Part print with two shaded views. Sizes in mm from the minimum x, y, z corner. Round coordinates to 2 decimals unless told otherwise and drop trailing zeros. Write each loop counter-clockwise with the first axis right and the second up, starting at its lowest first coordinate (ties: lowest second). Pieces come first, ordered by that corner, then holes. Notation, with made-up numbers: (35, -5) -> (88, -5) arc R29 cw to (88, 17) -> close; hole circle Ø10 at (45, 31). An arc over 180 degrees is marked (long way). Answer in a Markdown table with one row per item. Add a question column.
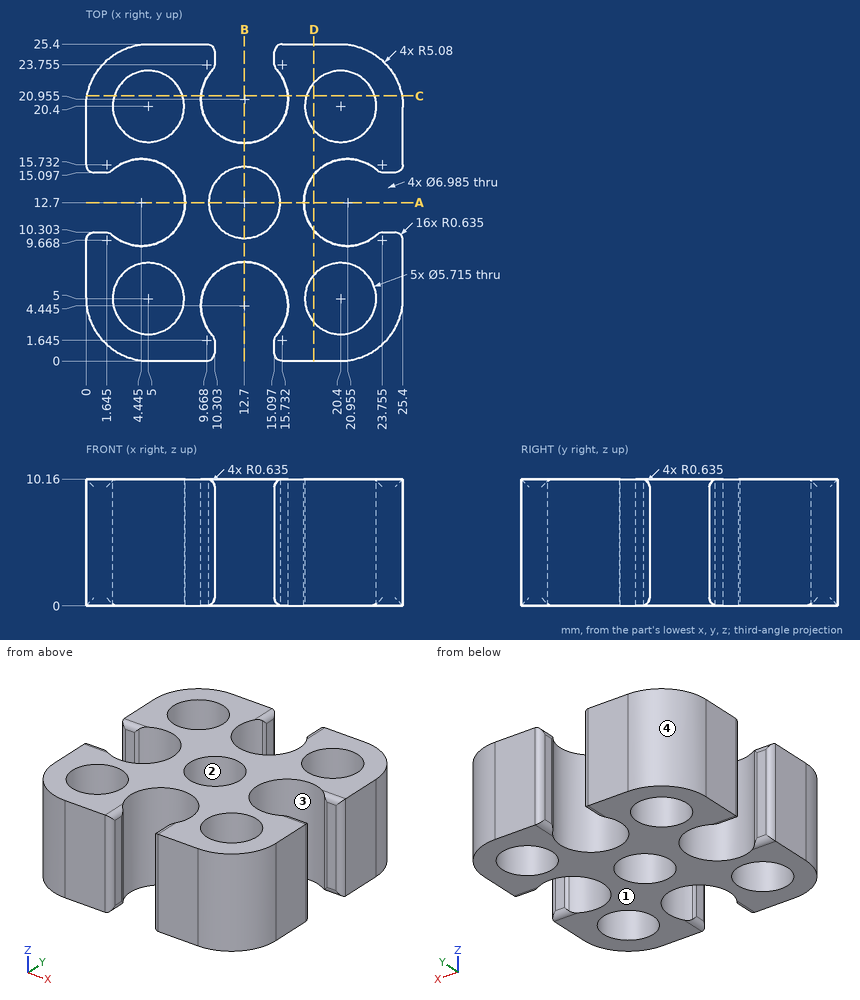
Item 1: Saw through at A-A on y = 12.7. Give the cut face in (x, z).
Item 2: Pin check, flat tips, straight feed: pin 1 (1.1 mm diameter, centred on y = 24.5, z = 6.5, fed in from +X) (1 decimal); pin 2 (11 mm diameter, centred on x = 12.7, y = 20.955, fed in from +Z); pin 3 (0.5 mm diameter, centred on y = 24, z = 5.5, fed in from -X); pin 4 (0.5 mm diameter, centred on x = 1, z = 7, fed in from +Y). Stop position of each tip, or through.
Item 3: Saw through at C-C on y = 21.25. Give the cut face in (x, z) (1 decimal).
Item 4: Saw through at D-D on x = 18.25. Give the cut face in (y, z).
Item 5: Drill centre lines: probe 1 along X at (y, z) = (3.75, 3.25); probe 2 along X at (y, z) = (21.25, 3.75) (1 decimal). Where is each one in solid material? Low to high.
Item 6: Two-plate mould, pull along X, no slides. Class the marked faces 1, 2, 3 and 4: +X half, -X half, draft (parallel to the pull), parting line (faces both ways), or undercut.
Recorded:
| question | item | result |
|---|---|---|
| 1 | outline | (7.94, 0) -> (9.84, 0) -> (9.84, 10.16) -> (7.94, 10.16) -> close; (15.56, 0) -> (17.46, 0) -> (17.46, 10.16) -> (15.56, 10.16) -> close |
| 2 | pin 1 | x = 23.9 |
| 2 | pin 2 | z = 10.16 |
| 2 | pin 3 | x = 1.33 |
| 2 | pin 4 | y = 23.66 |
| 3 | outline | (0.1, 0) -> (2.3, 0) -> (2.3, 10.2) -> (0.1, 10.2) -> close; (7.7, 0) -> (9.2, 0) -> (9.2, 10.2) -> (7.7, 10.2) -> close; (16.2, 0) -> (17.7, 0) -> (17.7, 10.2) -> (16.2, 10.2) -> close; (23.1, 0) -> (25.3, 0) -> (25.3, 10.2) -> (23.1, 10.2) -> close |
| 4 | outline | (0, 0) -> (3.12, 0) -> (3.12, 10.16) -> (0, 10.16) -> close; (6.88, 0) -> (10.49, 0) -> (10.49, 10.16) -> (6.88, 10.16) -> close; (14.91, 0) -> (18.52, 0) -> (18.52, 10.16) -> (14.91, 10.16) -> close; (22.28, 0) -> (25.4, 0) -> (25.4, 10.16) -> (22.28, 10.16) -> close |
| 5 | probe 1 | 0.18 to 2.43, 7.57 to 9.28, 16.12 to 17.83, 22.97 to 25.22 |
| 5 | probe 2 | 0.1 to 2.3, 7.7 to 9.2, 16.2 to 17.7, 23.1 to 25.3 |
| 6 | face 1 | draft |
| 6 | face 2 | undercut |
| 6 | face 3 | undercut |
| 6 | face 4 | -X half |
